Here's the drawing with two shaded views (mm, measured from the low corner). I have some questions. A direction names the side the tool comes from. Give positions to 0.01 mm unless a question says otherwise; leave off trailing zeros. Write each loop counter-clockwise with the first axis right and the second up, starting at its lowest first coordinate (ties: lowest second). Pieces come first, ordered by that corner, then holes.
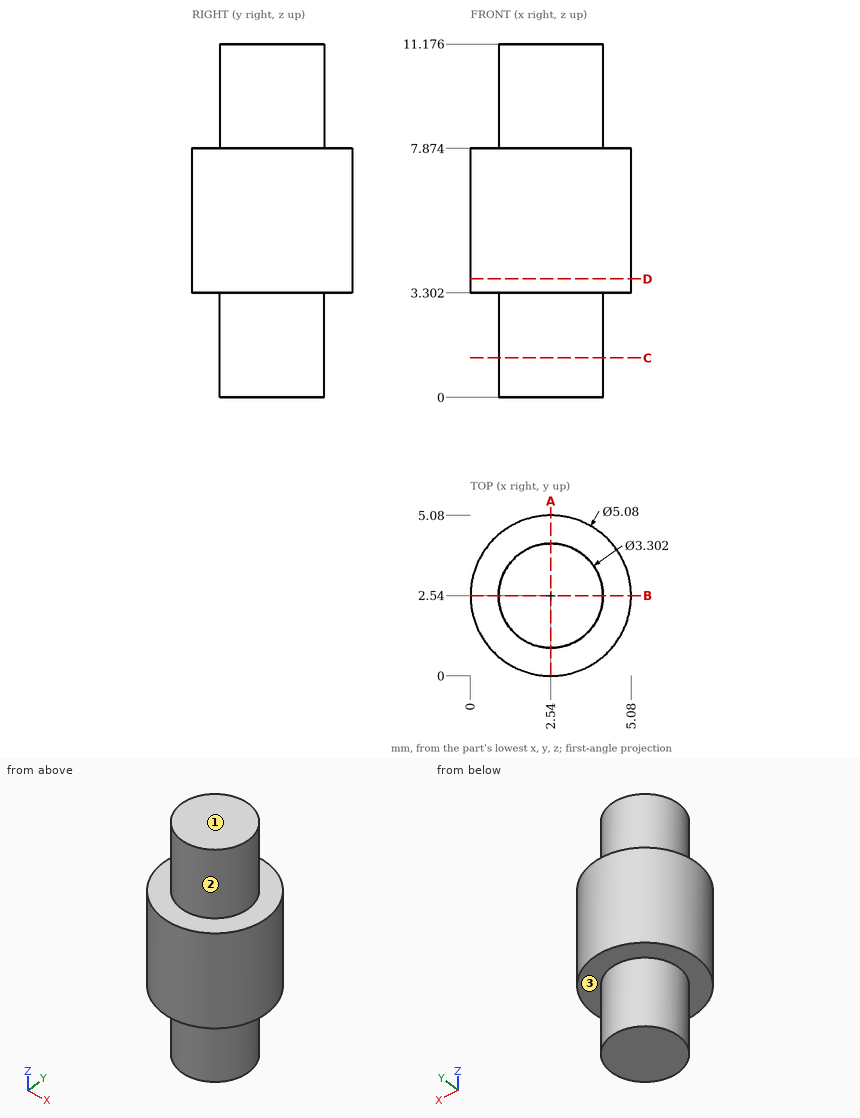
(1) For the marked faces 1, 2 and 3, which set-ups out of +Z, -Z, +X, -X, +Y, -Y let a thin tool reach every point of the face, with its end or its side?
Returned:
face 1: +Z, +X, -X, +Y, -Y
face 2: +Z
face 3: -Z
(2) Imagine slicing it at A-A, the plane x = 2.54. Write out the boundary of the cut face in (y, z).
Returned:
outline: (0, 3.3) - (0.89, 3.3) - (0.89, 0) - (4.19, 0) - (4.19, 3.3) - (5.08, 3.3) - (5.08, 7.87) - (4.19, 7.87) - (4.19, 11.18) - (0.89, 11.18) - (0.89, 7.87) - (0, 7.87) - close
(3) Imagine slicing it at D-D, the plane z = 3.75. Write out the boundary of the cut face in (x, y), plus the area to 3 significant figures.
Returned:
outline: circle Ø5.08 at (2.54, 2.54)
area: 20.3 mm2
(4) Will this pin go through, and if not, where does the flat tip stop? P1, Ø1, axis at x = 1.5, z = 3, coming from the +Y side.
Returned:
P1: stops at y = 5
(5) Imagine slicing it at C-C, the plane z = 1.25. Write out the boundary of the cut face in (x, y), plus the area to 3 significant figures.
Returned:
outline: circle Ø3.3 at (2.54, 2.54)
area: 8.56 mm2
(6) If I drill on L1, parallel to Z at x = 3.8, y = 3.9; L2, parallel to X at y = 2.5, z = 1.5; L3, parallel to X at y = 4.2, z = 5, over which ranges is the centre line in solid material (lowest first)?
Returned:
L1: z = 3.3 to 7.87
L2: x = 0.89 to 4.19
L3: x = 0.62 to 4.46
